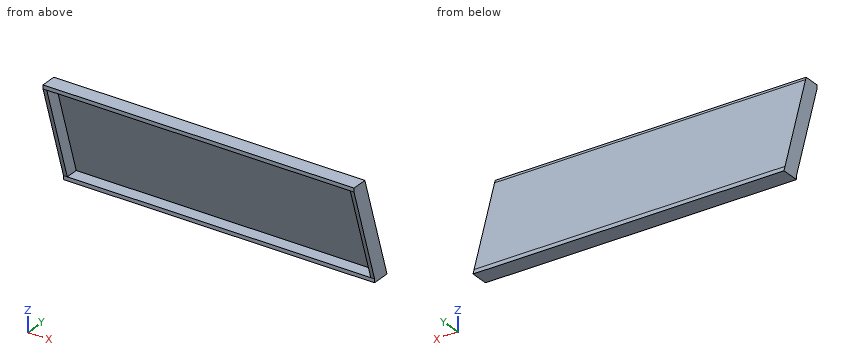
```python
from build123d import *

# Parameters (mm, degrees)
BOSS_EXTRUDE2_DEPTH = 166
BOSS_EXTRUDE3_DEPTH = 2
BOSS_EXTRUDE4_DEPTH = 2


with BuildPart() as part:
    # Sketch2 → Boss-Extrude2 (new body)
    with BuildSketch(Plane(origin=(0, 0, 0), x_dir=(0, 0, -1), z_dir=(1, 0, 0))):
        Polygon((51, -1.737908105), (51, -8.737908105), (53, -8.737908105), (53, -1.737908105), (53, 0.985657074), (50.401319851, 0.17038487), (-0.598680149, -15.82961513), (-2, -16.269244887), (-2, -17.737908105), (-2, -24.737908105), (0, -24.737908105), (0, -22.737908105), (0, -17.737908105), align=None)
    extrude(amount=BOSS_EXTRUDE2_DEPTH)

    # Sketch3 → Boss-Extrude3 (add)
    with BuildSketch(Plane.ZY):
        Polygon((-51, -1.737908105), (0, -17.737908105), (0, -24.737908105), (-51, -8.737908105), align=None)
    extrude(amount=-BOSS_EXTRUDE3_DEPTH)

    # Sketch4 → Boss-Extrude4 (add)
    with BuildSketch(Plane(origin=(166, 0, 0), x_dir=(0, 0, -1), z_dir=(1, 0, 0))):
        Polygon((51, -1.737908105), (0, -17.737908105), (0, -24.737908105), (51, -8.737908105), align=None)
    extrude(amount=-BOSS_EXTRUDE4_DEPTH)


solid = part.part
```
Geometry check sheet. Reference: the model listing, model coordinates, mm. Give positions to 0.01 mm unless a question says otherwise; leave off trailing zeros. Order: outer loops, then holes, each group sorted by start corner. A loop starts at its lowest first (then second) coordinate and runs counter-clockwise, first axis right, second up. Notation, with made-up numbers: (-34.75, 11.5) - (10.25, 11.5) arc R18 cw to (10.25, 25.5) - close; hole circle Ø4 at (-29, -30.5). An arc over 180 degrees is marked (long way). Answer in a Markdown table with one row per item. Add a question column.
Q1. Cross-section at C-C, the plane z = -26.5. Enter the section's corners in (x, y), then the cut area to 3 significant figures.
Q2. Cross-section at B-B, the plane y = -4.5. Enter the section's corners in (x, z), then the cut area to 3 significant figures.
Q3. Material ranges on probe 1 along X at (y, z) = (-19.25, -9); probe 2 along Z at (x, y) = (109, -21.75); probe 3 along Y at (x, z) = (81.5, -39), recorded low to high. Write a range as from..to.
Q4. Cross-section at D-D, the plane y = -19.5. Enter the section's corners in (x, z), then the cut area to 3 significant figures.
Q5. Gauge pin test, flat ends, axial feed: pin 1 (5.5 mm diameter, centred on x = 80, y = -21.5, fed in from -Z); pin 2 (1.6 mm diameter, centred on x = 119, z = -52, fed in from -Y); pin 3 (1 mm diameter, centred on x = 41.5, z = -31.5, fed in from -Y). Record the tip position at first contact, or that the pin passes through.
Q6. Cross-section at A-A, the plane x = 125. Enter the section's corners in (y, z).
Check values:
| question | item | result |
|---|---|---|
| 1 | outline | (0, -16.42) - (2, -16.42) - (2, -9.42) - (164, -9.42) - (164, -16.42) - (166, -16.42) - (166, -7.33) - (0, -7.33) - close |
| 1 | area | 376 mm^2 |
| 2 | outline | (0, -53) - (166, -53) - (166, -35.51) - (0, -35.51) - close; hole (2, -51) - (164, -51) - (164, -42.2) - (2, -42.2) - close |
| 2 | area | 1,480 mm^2 |
| 3 | probe 1 | x = 0..2, 164..166 |
| 3 | probe 2 | z = 0..2 |
| 3 | probe 3 | y = -5.5..-3.41 |
| 4 | outline | (0, -16.7) - (2, -16.7) - (2, 0) - (164, 0) - (164, -16.7) - (166, -16.7) - (166, 2) - (0, 2) - close |
| 4 | area | 399 mm^2 |
| 5 | pin 1 | stops at z = 0 |
| 5 | pin 2 | stops at y = -8.74 |
| 5 | pin 3 | stops at y = -8.01 |
| 6 | outline | (-24.74, 0) - (-17.74, 0) - (-1.74, -51) - (-8.74, -51) - (-8.74, -53) - (0.99, -53) - (-16.27, 2) - (-24.74, 2) - close |
